Read the model definition and answer for the solid it produces. Units are mm, in the model's axes. Face numbers are marked on the shaded views. A direction names the side the tool comes from. Give positions to 0.01 mm unless a question says otherwise; leave off trailing zeros. Write each loop counter-clockwise with the first axis right and the second up, starting at its lowest first coordinate (ties: lowest second). Pieces come first, ordered by that corner, then holes. Notation, with made-up numbers: (-30, 68.25) -> (-15, 68.25) arc R28 cw to (-15, 107.25) -> close; hole circle Ø1 at (-36, -22.75). An arc over 180 degrees is marked (long way). Answer as CSV lines item,"result". Start each with the question number.
1. Find the intervals of material crossed by line 1 (Y direction, x = 22.5, z = 1.5); line 2 (X direction, y = -4.5, z = 7.5); line 3 (X direction, y = -3.75, z = 4.5), in increasing order.
2. The part is cut by section C-C, the plane z = 20. Determine the outline of the cut face in (x, y).
3. A tool of negligible diameter and unlimited length cuts with its end or side. For the marked faces 1, 2 and 3, from which of +Z, -Z, +X, -X, +Y, -Y can it reach the whole face along a straight path? Write none if from no direction.
4. Given pin 1 (9 mm diameter, centred on x = 13, z = 18, fed in from -Y); pin 2 (10 mm diameter, centred on x = 19, z = 7, fed in from +Y); pin 3 (4 mm diameter, centred on y = -4, z = 5, fed in from +X), each flat-ended and moving along its own axis, determine where each tip first touches the part or whether it passes through.
5. The part is cut by section D-D, the plane x = 28.5. Determine the outline of the cut face in (y, z), and give its area (3 significant figures).
6. The part is cut by section B-B, the plane x = -22.5. Determine the outline of the cut face in (y, z), and give its area (3 significant figures).
7. The part is cut by section A-A, the plane y = -3.75. Determine the outline of the cut face in (x, z).
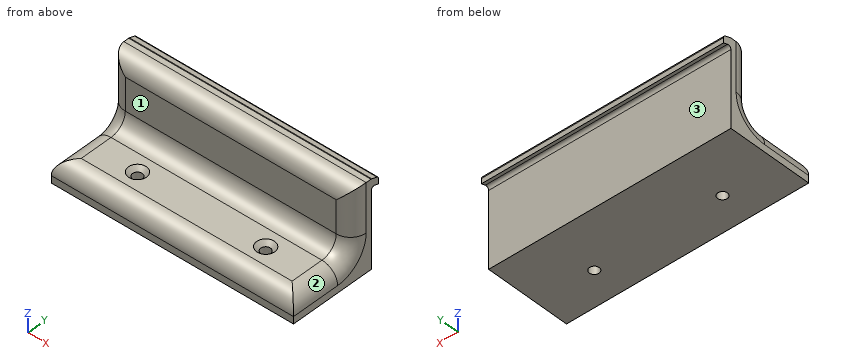
from build123d import *

# Parameters (mm, degrees)
SKETCH1_W                                       = 85
SKETCH1_H                                       = 30
BOSS_EXTRUDE1_DEPTH                             = 8
SKETCH2_W                                       = 85
SKETCH2_H                                       = 7.5
BOSS_EXTRUDE2_DEPTH                             = 22.5
CSK_FOR_M3_FLAT_HEAD_MACHINE_SCREW1_D           = 3.4
CSK_FOR_M3_FLAT_HEAD_MACHINE_SCREW1_CSINK_D     = 6.3
CSK_FOR_M3_FLAT_HEAD_MACHINE_SCREW1_CSINK_ANGLE = 90
BOSS_EXTRUDE3_DEPTH                             = 85
FILLET1_R                                       = 5.5
FILLET2_R                                       = 1
FILLET3_R                                       = 1


with BuildPart() as part:
    # Sketch1 → Boss-Extrude1 (new body)
    with BuildSketch(Plane.XY):
        Rectangle(SKETCH1_W, SKETCH1_H)
    extrude(amount=BOSS_EXTRUDE1_DEPTH)

    # Sketch2 → Boss-Extrude2 (add)
    with BuildSketch(Plane.XY.offset(8)):
        with Locations((0, 11.25)):
            Rectangle(SKETCH2_W, SKETCH2_H)
    extrude(amount=BOSS_EXTRUDE2_DEPTH)

    # CSK for M3 Flat Head Machine Screw1 (through all)
    with Locations(Plane.XY.offset(8)):
        with Locations((-22.5, -3.75), (22.5, -3.75)):
            CounterSinkHole(CSK_FOR_M3_FLAT_HEAD_MACHINE_SCREW1_D / 2, CSK_FOR_M3_FLAT_HEAD_MACHINE_SCREW1_CSINK_D / 2, counter_sink_angle=CSK_FOR_M3_FLAT_HEAD_MACHINE_SCREW1_CSINK_ANGLE)

    # Sketch7 → Boss-Extrude3 (add)
    with BuildSketch(Plane.ZY.offset(42.5)):
        Polygon((30.5, 15), (29.572949017, 17.853169549), (27.072949017, 17.853169549), (28, 15), align=None)
    extrude(amount=-BOSS_EXTRUDE3_DEPTH)

    # Fillet1
    fillet1_edges = [part.edges().sort_by_distance(p)[0] for p in [
        (0, -15, 8),
        (-42.5, -3.75, 8),
        (0, 7.5, 8),
        (-42.5, 7.5, 19.25),
        (42.5, 7.5, 19.25),
        (0, 7.5, 30.5),
        (42.5, -3.75, 8),
    ]]
    fillet(fillet1_edges, radius=FILLET1_R)

    # Fillet2
    fillet2_edges = [part.edges().sort_by_distance(p)[0] for p in [
        (0, 15, 28),
    ]]
    fillet(fillet2_edges, radius=FILLET2_R)

    # Fillet3
    fillet3_edges = [part.edges().sort_by_distance(p)[0] for p in [
        (0, 15, 30.5),
        (0, 17.853169549, 29.572949017),
    ]]
    fillet(fillet3_edges, radius=FILLET3_R)


solid = part.part
Results found:
1,line 1,"y = -15 to -5.45, -2.05 to 15"
1,line 2,"x = -39.29 to -25.04, -19.96 to 19.96, 25.04 to 39.29"
1,line 3,"x = -42.12 to -24.2, -20.8 to 20.8, 24.2 to 42.12"
2,outline,"(-42.5, 13) arc R5.5 ccw to (-37, 7.5) -> (37, 7.5) arc R5.5 ccw to (42.5, 13) -> (42.5, 15) -> (-42.5, 15) -> close"
3,face 1,"+Z, +X, -X, -Y"
3,face 2,"+Z, +X, -Y"
3,face 3,"-Z, +X, -X, +Y"
4,pin 1,"stops at y = 7.5"
4,pin 2,"stops at y = 15"
4,pin 3,"stops at x = 42.48"
5,outline,"(-15, 0) -> (15, 0) -> (15, 26.62) arc R1 cw to (16.31, 27.57) -> (17.85, 27.07) -> (17.85, 28.85) arc R1 ccw to (17.16, 29.8) -> (15.15, 30.45) arc R1 ccw to (14.84, 30.5) -> (13, 30.5) arc R5.5 ccw to (7.5, 25) -> (7.5, 13.5) arc R5.5 cw to (2, 8) -> (-9.5, 8) arc R5.5 ccw to (-15, 2.5) -> close"
5,area,"410 mm²"
6,outline,"(-15, 0) -> (-5.45, 0) -> (-5.45, 6.55) -> (-6.9, 8) -> (-9.5, 8) arc R5.5 ccw to (-15, 2.5) -> close; (-2.05, 0) -> (15, 0) -> (15, 26.62) arc R1 cw to (16.31, 27.57) -> (17.85, 27.07) -> (17.85, 28.85) arc R1 ccw to (17.16, 29.8) -> (15.15, 30.45) arc R1 ccw to (14.84, 30.5) -> (13, 30.5) arc R5.5 ccw to (7.5, 25) -> (7.5, 13.5) arc R5.5 cw to (2, 8) -> (-0.6, 8) -> (-2.05, 6.55) -> close"
6,area,"380 mm²"
7,outline,"(-42.5, 0) -> (-24.2, 0) -> (-24.2, 6.55) -> (-25.65, 8) -> (-37, 8) arc R5.5 ccw to (-42.5, 2.5) -> close; (-20.8, 0) -> (20.8, 0) -> (20.8, 6.55) -> (19.35, 8) -> (-19.35, 8) -> (-20.8, 6.55) -> close; (24.2, 0) -> (42.5, 0) -> (42.5, 2.5) arc R5.5 ccw to (37, 8) -> (25.65, 8) -> (24.2, 6.55) -> close"
